CAD build for the part. Positions are in the model's coordinates, mm. Face numbers are marked on the shaded views. A direction names the side the tool comes from. Coordinates: 2 decimals unless noted, no trailing zeros. Loops run counter-clockwise (first coordinate to the right, second up) from the corner with the lowest first, then second, coordinate; pieces in that order, holes last. Notation, with made-up numbers: (6, 21.5) -> (56, 21.5) arc R17 ccw to (56, 33.5) -> close; hole circle Ø6 at (-35.75, 65). An arc over 180 degrees is marked (long way). Return JSON: item names as keys, results as strings. Group by question number.
(1) Saw through at A-A on x = 2. Write the cut outline in (y, z), then the cut area to 3 significant figures.
(2) Saw through at C-C on x = 14.5. Write the cut outline in (y, z), then the cut area to 3 significant figures.
(3) Tool access for the marked faces 1, 2 and 3: list every direction of +Z, -Z, +X, -X, +Y, -Y with a clear straight run to the whole face (end or side of a thin tool).
(4) Probe L1, parallel to X at y = 6, z = -1; L2, parallel to X at y = -0.25, z = 5.5; L3, parallel to Z at x = -4, y = -4. List the from-to ranges inside material, lowest first.
(5) Saw through at B-B on x = -2. Write the cut outline in (y, z).
(6) Flat gauge pins, fed straight in: pin 1 Ø6 at (x, y) = (17.5, -1) entering from +Z; pin 2 Ø5 at (x, y) = (6.5, -5) entering from +Z; pin 3 Ø1.5 at (x, z) = (4.5, 2.5) entering from +Y. Where does each tip first touch, or does it go through?
Autodesk Inventor part; units mm, degrees
ref_plane "YZ Plane" through (0, 0, 0) normal (1, 0, 0) x (0, 1, 0)
ref_plane "XZ Plane" through (0, 0, 0) normal (0, 1, 0) x (-1, 0, 0)
ref_plane "XY Plane" through (0, 0, 0) normal (0, 0, 1) x (1, 0, 0)
sketch "Skizze1" plane through (0, 0, 0) normal (0, 0, 1) x (1, 0, 0)
  line L0 (0, 5.7) -> (0, 3.6617)
  line L1 (3.75, 4) -> (25, 4)
  line L2 (25, 4) -> (25, 0)
  line L3 (25, 0) -> (-0.6001, 0)
  line L4 (-0.4751, 0) -> (2.675, 0)
  line L5 (-0.6001, 0) -> (-0.6001, 5.7)
  line L6 (-0.6001, 5.7) -> (0, 5.7)
  line L7 (3.75, 4) -> (2.9831, 3.6617)
  line L8 (2.9831, 3.6617) -> (0, 3.6617)
  line L9 (0, -0.1135) -> (0, 1.4755)
  dimension "d0" = 25
  dimension "d1" = 21.25
  dimension "d2" = 8
  dimension "d9" = 0.6001
  dimension "d10" = 11.4
  dimension "d13" = 0.7669
  dimension "d14" = 7.3234
revolve "Körper" add sketch "Skizze1" angle 360 about axis through (25, 0, 0) along (-1, 0, 0)
sketch "Skizze2" plane through (-0.6001, 0, 0) normal (-1, 0, 0) x (0, 0, 1)
  line L0 (0, 7.5056) -> (6.5, 3.7528)
  line L1 (6.5, 3.7528) -> (6.5, -3.7528)
  line L2 (6.5, -3.7528) -> (0, -7.5056)
  line L3 (0, -7.5056) -> (-6.5, -3.7528)
  line L4 (-6.5, -3.7528) -> (-6.5, 3.7528)
  line L5 (-6.5, 3.7528) -> (0, 7.5056)
  point P0 (0, 0)
  point P1 (0, 0)
  dimension "d11" = 13
extrude "Kopf" add sketch "Skizze2" along normal blind 4.7
sketch "Skizze4" plane through (0, 0, 0) normal (0, 0, 1) x (1, 0, 0)
  line L0 (-5.3001, 6.5) -> (-5.3001, 7.5056)
  line L1 (-5.3001, 7.5056) -> (-4.7195, 7.5056)
  line L2 (-4.7195, 7.5056) -> (-5.3001, 6.5)
  line L3 (-1.1851, 0) -> (0.0049, 0)
  line L4 (-0.6001, 7.5056) -> (-5.3001, 7.5056)
  line L5 (-5.3001, 3.7528) -> (-5.3001, 7.5056)
  dimension "d5" = 30
  dimension "d19" = 13
revolve "Fase1" cut sketch "Skizze4" angle 360 about axis through (-10, 0, 0) along (1, 0, 0)
thread "Gewinde"
chamfer "Fase2" distance 0.7668 distance2 0.7669 1 edges at (25, -4, 0) measured on face at (25, 0.998, -0.8842)
equation "\"d0\" = NLG"
equation "\"d1\" = GEL"
equation "\"d2\" = GD"
equation "\"d10\" = SD2"
equation "\"d14\" = BDM"
equation "\"d11\" = SW"
equation "\"d3\" = KOH - SD"
equation "\"d5\" = ANG1"
equation "\"d19\" = SW0"
equation "\"d15\" = GEL"
equation "\"d6\" = -0.5 * SPD + 0.5 * GD"
equation "\"NLG\" = 25"
equation "\"GD\" = NND"
equation "\"BDM\" = 7.32342"
equation "\"KOH\" = 5.3"
equation "\"GEL\" = 21.25"
equation "\"SW\" = 13"
equation "\"SW0\" = 13"
equation "\"SPD\" = NND - 1.2269 * TPU"
equation "\"SD2\" = 11.4"
equation "\"SD\" = 0.6"
equation "\"ANG1\" = 30deg"
equation "\"GAL\" = 0.61345 * TPU"
equation "\"GUL\" = 0.61345 * TPU"
equation "\"RR\" = 0.4"
equation "\"d20\" = -NLG"
equation "\"TOA\" = 30deg"
equation "\"PTC\" = TPU"
equation "\"GD1\" = THREADDIA - 1.2269 * TPU"
equation "\"TPU\" = 1.25"
equation "\"THREADDIA\" = 8"
equation "\"E0\" = 1.155 * SW"
equation "\"NND\" = 8"
properties part number "DIN 933 - M8  x 25"
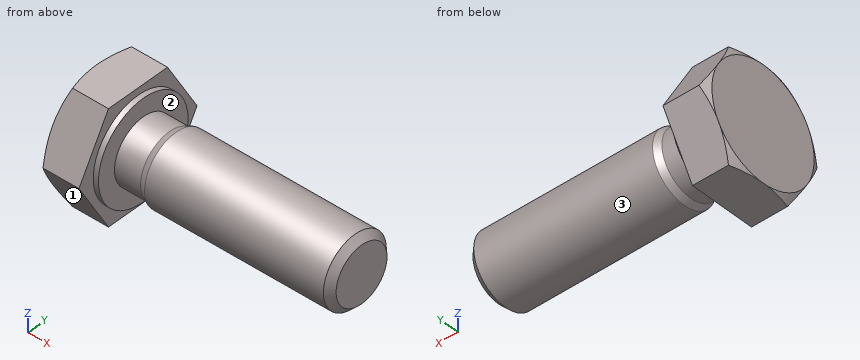
Geometry results:
{
 "1": {"outline": "circle Ø7.32 at (0, 0)", "area": "42.1 mm²"},
 "2": {"outline": "circle Ø8 at (0, 0)", "area": "50.3 mm²"},
 "3": {"face 1": "-Z, +X, -X, -Y", "face 2": "none", "face 3": "+X"},
 "4": {"L1": "-5.3 to -0.6", "L2": "-5.3 to 0", "L3": "-6.07 to 6.07"},
 "5": {"outline": "(-7.51, 0) -> (-3.75, -6.5) -> (3.75, -6.5) -> (7.51, 0) -> (3.75, 6.5) -> (-3.75, 6.5) -> close"},
 "6": {"pin 1": "z = 4", "pin 2": "z = 3.12", "pin 3": "y = 3.6"}
}
